from build123d import *

# Parameters (mm, degrees)
EXTRUDE_1_DEPTH     = 50
EXTRUDE_2_DEPTH     = 3
EXTRUDE_START       = -3
EXTRUDE_3_DEPTH     = 3
SKETCH_5_R          = 11
SKETCH_5_R_2        = 1.75
CUT_EXTRUDE_1_DEPTH = 3
CUT_EXTRUDE_2_DEPTH = 11
CHAMFER_1_SIZE      = 5


with BuildPart() as part:
    # 草图1 → 凸台-拉伸1 (new body)
    with BuildSketch(Plane(origin=(0, 0, 0), x_dir=(0, 0, -1), z_dir=(1, 0, 0))):
        with BuildLine():
            Line((0, 2), (0, 51))
            Line((0, 51), (3, 51))
            Line((3, 51), (3, 5))
            ThreePointArc((3, 5), (3.585786438, 3.585786438), (5, 3))
            Line((5, 3), (53, 3))
            Line((53, 3), (53, 0))
            Line((53, 0), (2, 0))
            ThreePointArc((2, 0), (0.585786438, 0.585786438), (0, 2))
        make_face()
    extrude(amount=EXTRUDE_1_DEPTH)

    # 草图3 → 凸台-拉伸2 (add)
    with BuildSketch(Plane(origin=(0, 0, 0), x_dir=(0, 0, -1), z_dir=(1, 0, 0))):
        with BuildLine():
            Line((3, 5), (3, 23))
            Line((3, 23), (16, 3))
            Line((16, 3), (5, 3))
            ThreePointArc((5, 3), (3.585786438, 3.585786438), (3, 5))
        make_face()
    extrude(amount=EXTRUDE_2_DEPTH)

    # 草图4 → 凸台-拉伸3 (add)
    with BuildSketch(Plane(origin=(50, 0, 0), x_dir=(0, 0, -1), z_dir=(1, 0, 0)).offset(EXTRUDE_START)):
        with BuildLine():
            Line((3, 23), (3, 5))
            ThreePointArc((3, 5), (3.585786438, 3.585786438), (5, 3))
            Line((5, 3), (16, 3))
            Line((16, 3), (3, 23))
        make_face()
    extrude(amount=EXTRUDE_3_DEPTH)

    # 草图5 → 切除-拉伸1 (cut)
    with BuildSketch(Plane.XY):
        with Locations((25, 30)):
            Circle(SKETCH_5_R)
        with Locations((9.5, 45.5)):
            Circle(SKETCH_5_R_2)
        with Locations((40.5, 45.5)):
            Circle(SKETCH_5_R_2)
        with Locations((9.5, 14.5)):
            Circle(SKETCH_5_R_2)
        with Locations((40.5, 14.5)):
            Circle(SKETCH_5_R_2)
    extrude(amount=-CUT_EXTRUDE_1_DEPTH, mode=Mode.SUBTRACT)

    # 草图6 → 切除-拉伸2 (cut)
    with BuildSketch(Plane(origin=(0, 0, 0), x_dir=(1, 0, 0), z_dir=(0, 1, 0))):
        with BuildLine():
            Line((7.9, 41.5), (7.9, 11.5))
            ThreePointArc((7.9, 11.5), (10, 9.4), (12.1, 11.5))
            Line((12.1, 11.5), (12.1, 41.5))
            ThreePointArc((12.1, 41.5), (10, 43.6), (7.9, 41.5))
        make_face()
        with BuildLine():
            Line((37.9, 41.5), (37.9, 11.5))
            ThreePointArc((37.9, 11.5), (40, 9.4), (42.1, 11.5))
            Line((42.1, 11.5), (42.1, 41.5))
            ThreePointArc((42.1, 41.5), (40, 43.6), (37.9, 41.5))
        make_face()
    extrude(amount=CUT_EXTRUDE_2_DEPTH, mode=Mode.SUBTRACT)

    # 倒角1
    chamfer_1_edges = [part.edges().sort_by_distance(p)[0] for p in [
        (0, 51, -1.5),
        (50, 1.5, -53),
        (50, 51, -1.5),
        (0, 1.5, -53),
    ]]
    chamfer(chamfer_1_edges, length=CHAMFER_1_SIZE)


solid = part.part
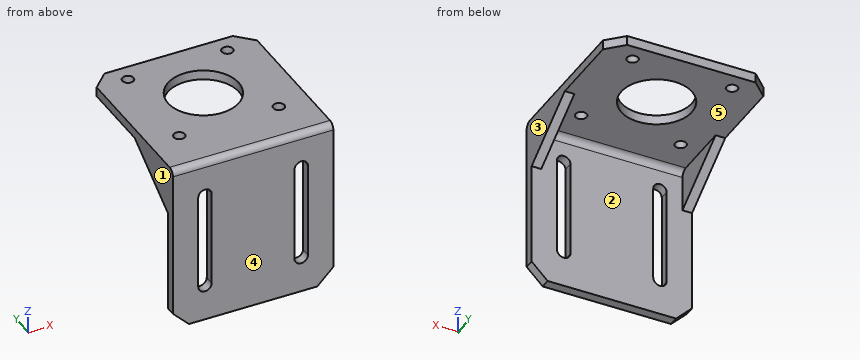
Part model, mm, in its own coordinate system. Face numbers are marked on the shaded views. A direction names the side the tool comes from. Give positions to 0.01 mm unless a question says otherwise; leave off trailing zeros. Loops run counter-clockwise (first coordinate to the right, second up) from the corner with the lowest first, then second, coordinate; pieces in that order, holes last. Notation, with made-up numbers: M 13,83.25 L 55,83.25 A15 ccw 55,87.25 Z; hole C -10.5,-20 d5. An arc over 180 degrees is marked long. Put each result on its own line as item: value. Start each with the question number.
1) Saw through at B-B (y = 25). List the corners of the cut face in (x, z).
2) 3-axis set-ups, long thin cutter, end or side, ignore diameter. For the marked faces 4 and 5: which of +Z, -Z, +X, -X, +Y, -Y reach the whole face in a straight line?
3) Pull direction X, two halves, no side cores. Call the marked faces 1, 2 and 3: +X half, -X half, draft (parallel to the pull), parting line (faces both ways), or undercut.
4) Saw through at A-A (z = -25). List the corners of the cut face in (x, y).
5) Probe probe 1 along X at (y, z) = (14, -1); probe 2 along Y at (x, z) = (30.5, -28); probe 3 along Y at (x, z) = (25, -1.9). List the from-to ranges inside material, lowest first.
6) Saw through at C-C (x = 40.5). List the corners of the cut face in (y, z).
7) Saw through at D-D (y = 14.5). List the corners of the cut face in (x, z) (3 decimals).
8) Flat gauge pins, fed straight in: pin 1 (17.5 mm diameter, centred on x = 25, y = 30, fed in from +Z); pin 2 (14 mm diameter, centred on x = 17, y = 38.5, fed in from -Z); pin 3 (10.5 mm diameter, centred on y = 13, z = -11.5, fed in from -X). Where does each tip first touch, or does it go through?
Numbers:
1. outline: M 0,-3 L 15.2,-3 L 15.2,0 L 0,0 Z; M 34.8,-3 L 50,-3 L 50,0 L 34.8,0 Z
2. face 4: +Z, -Z, +X, -X, -Y
2. face 5: -Z, +Y
3. face 1: -X half
3. face 2: undercut
3. face 3: +X half
4. outline: M 0,0 L 7.9,0 L 7.9,3 L 0,3 Z; M 12.1,0 L 37.9,0 L 37.9,3 L 12.1,3 Z; M 42.1,0 L 50,0 L 50,3 L 42.1,3 Z
5. probe 1: 0 to 7.82, 11.18 to 38.82, 42.18 to 50
5. probe 2: 0 to 3
5. probe 3: 0 to 19, 41 to 51
6. outline: M 0,-53 L 3,-53 L 3,-43.54 L 0,-43.54 Z; M 0,-9.46 L 3,-9.46 L 3,-5 A2 cw 5,-3 L 12.75,-3 L 12.75,0 L 2,0 A2 ccw 0,-2 Z; M 16.25,-3 L 43.75,-3 L 43.75,0 L 16.25,0 Z; M 47.25,-3 L 51,-3 L 51,0 L 47.25,0 Z
7. outline: M 0,-8.525 L 3,-8.525 L 3,-3 L 7.75,-3 L 7.75,0 L 0,0 Z; M 11.25,-3 L 38.75,-3 L 38.75,0 L 11.25,0 Z; M 42.25,-3 L 47,-3 L 47,-8.525 L 50,-8.525 L 50,0 L 42.25,0 Z
8. pin 1: through
8. pin 2: z = -3
8. pin 3: x = 0
